Read the model definition and answer for the solid it produces. Units are mm, in the model's axes. A direction names the side the tool comes from. Give positions to 0.01 mm unless a question says otherwise; leave off trailing zeros. Loops run counter-clockwise (first coordinate to the right, second up) from the corner with the lowest first, then second, coordinate; pieces in that order, holes last. Notation, with made-up numbers: (-21.75, -27) - (-14.75, -27) arc R13 ccw to (-14.75, -19) - close; hole circle Ø11 at (78, 39). An arc over 180 degrees is marked (long way). Put each result on its own line as item: value. Start each with the question number.
1. For a pull along Y with two mould halves and no side action, classify faces 1 (the flat face through (7.3, 11.46, -2.3)), 2 (the flat face through (-4, 6.46, 5)), 3 (the cylindrical face through (-6, 38, 0)) as released by +Y, released by -Y, zero draft, split by the parting line, or undercut.
2. For faces 4 (the cylindrical face through (-0.867, 0.39, 3.905)), 5 (the flat face through (0, 29, 7.794)), 6 (the flat face through (4, 31.96, 5)), determine the directions among +Z, -Z, +X, -X, +Y, -Y from which every point of the face is accessible in a straight line to the end or side of a thin tool.
3. A cutting plane is placed at A-A, the plane y = 28. Determine the outline of the cut face in (x, z), plus the area to 3 significant figures.
4. Given pin 1 Ø2 at (y, z) = (26.5, 3.5) entering from -X; pin 2 Ø7 at (x, z) = (0, 0) entering from -Y; pin 3 Ø4 at (x, z) = (0.5, -1) entering from +Y, each flat-ended and moving along its own axis, determine where each tip first touches the part or whether it passes through.
5. A cutting plane is placed at B-B, the plane z = 6.5. Determine the outline of the cut face in (x, y), plus the area to 3 significant figures.
6. A cutting plane is placed at C-C, the plane y = 18.5. Determine the outline of the cut face in (x, z), plus the area to 3 significant figures.
7. Consider L1, parallel to Z at x = 0, y = 12; L2, parallel to Z at x = 0, y = 35.25. Determine where each line is inside the solid, lowest interval first. Write a range as from..to.
```python
from build123d import *

# Parameters (mm, degrees)
CUT_EXTRUDE_1_DEPTH = 30


with BuildPart() as part:
    # Эскиз2 → Повернуть1 (revolve)
    with BuildSketch(Plane.XY):
        Polygon((4, -4.539806968), (6, -4.539806968), (6, 6.460193032), (9, 6.460193032), (9, 11.460193032), (7.5, 11.460193032), (7.5, 26.960193032), (9, 26.960193032), (9, 31.960193032), (6, 31.960193032), (6, 42.960193032), (4, 42.960193032), (4, 32.960193032), (2.5, 32.960193032), (2.5, 23.960193032), (0, 23.960193032), (0, 15.460193032), (2.5, 15.460193032), (2.5, 5.460193032), (4, 5.460193032), align=None)
    revolve(axis=Axis((0, 15.460193032, 0), (0, 1, 0)))

    # Эскиз3 → Вырез-Вытянуть1 (cut)
    with BuildSketch(Plane(origin=(0, 31.960193032, 0), x_dir=(1, 0, 0), z_dir=(0, 1, 0))):
        with BuildLine():
            Line((-9, 0), (-4.5, 7.794228634))
            ThreePointArc((-4.5, 7.794228634), (-7.794228634, 4.5), (-9, 0))
        make_face()
        with BuildLine():
            Line((-4.5, 7.794228634), (4.5, 7.794228634))
            ThreePointArc((4.5, 7.794228634), (0, 9), (-4.5, 7.794228634))
        make_face()
        with BuildLine():
            Line((4.5, 7.794228634), (9, 0))
            ThreePointArc((9, 0), (7.794228634, 4.5), (4.5, 7.794228634))
        make_face()
        with BuildLine():
            ThreePointArc((4.5, -7.794228634), (7.794228634, -4.5), (9, 0))
            Line((9, 0), (4.5, -7.794228634))
        make_face()
        with BuildLine():
            ThreePointArc((-4.5, -7.794228634), (0, -9), (4.5, -7.794228634))
            Line((4.5, -7.794228634), (-4.5, -7.794228634))
        make_face()
        with BuildLine():
            ThreePointArc((-9, 0), (-7.794228634, -4.5), (-4.5, -7.794228634))
            Line((-4.5, -7.794228634), (-9, 0))
        make_face()
    extrude(amount=-CUT_EXTRUDE_1_DEPTH, mode=Mode.SUBTRACT)


solid = part.part
```
Return value:
1. face 1: undercut
1. face 2: released by -Y
1. face 3: zero draft
2. face 4: -Y
2. face 5: +Z, +X, -X, +Y, -Y
2. face 6: +Y
3. outline: (-9, 0) - (-4.5, -7.79) - (4.5, -7.79) - (9, 0) - (4.5, 7.79) - (-4.5, 7.79) - close; hole circle Ø5 at (0, 0)
3. area: 191 mm2
4. pin 1: stops at x = -7.49
4. pin 2: stops at y = 5.46
4. pin 3: stops at y = 32.96
5. outline: (-5.25, 6.46) - (5.25, 6.46) - (5.25, 11.46) - (3.74, 11.46) - (3.74, 26.96) - (5.25, 26.96) - (5.25, 31.96) - (-5.25, 31.96) - (-5.25, 26.96) - (-3.74, 26.96) - (-3.74, 11.46) - (-5.25, 11.46) - close
5. area: 221 mm2
6. outline: circle Ø15 at (0, 0)
6. area: 177 mm2
7. L1: z = -7.5..-2.5, 2.5..7.5
7. L2: z = -6..-4, 4..6
